CAD build for the part. Positions are in the model's coordinates, mm. Face numbers are marked on the shaded views. A direction names the side the tool comes from. Give positions to 0.01 mm unless a question says otherwise; leave off trailing zeros. Write each loop counter-clockwise with the first axis right and the second up, starting at its lowest first coordinate (ties: lowest second). Pieces come first, ordered by that corner, then holes. Notation, with made-up numbers: (-3.75, -26) - (23.25, -26) arc R16 ccw to (23.25, 5) - close; hole circle Ø9 at (6.25, 55). An arc over 180 degrees is marked (long way). Answer as a JSON object with one key per item and string values.
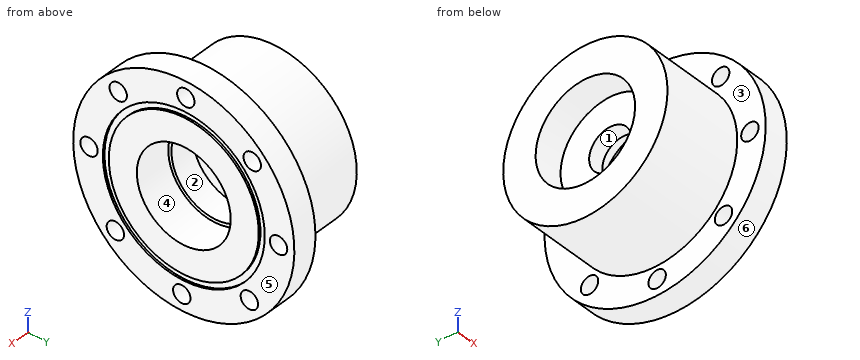
from build123d import *

# Parameters (mm, degrees)
M6_CLEARANCE_HOLE1_D = 7


with BuildPart() as part:
    # Main sketch → Revolve1 (revolve)
    with BuildSketch(Plane.XY, mode=Mode.PRIVATE) as revolve1_sk:
        Polygon((0, 8.500000018), (0, 20.000000005), (-11.999999876, 20.000000005), (-11.999999876, 33.02), (21.59, 33.02), (21.59, 44.45), (31.75, 44.45), (31.75, 32.54375), (30.972125, 32.54375), (30.972125, 30.1625), (31.75, 30.1625), (31.75, 18.8722), (16.6116, 18.8722), (16.6116, 17.6022), (6.35, 17.6022), (6.35, 8.500000018), align=None)
    revolve(revolve1_sk.sketch.rotate(Axis((71.950113838, 0, 0), (-1, 0, 0)), 90), axis=Axis((71.950113838, 0, 0), (-1, 0, 0)))

    # M6 Clearance Hole1 (through all)
    with Locations(Plane(origin=(31.75, 0, 0), x_dir=(0, 0, -1), z_dir=(1, 0, 0))):
        with Locations((0, 0), (-38.091322418, 0.813115257), (-27.509591698, -26.359673074), (-0.813115257, -38.091322418), (26.359673074, -27.509591698), (38.091322418, -0.813115257), (27.509591698, 26.359673074), (0.813115257, 38.091322418), (-26.359673074, 27.509591698)):
            Hole(M6_CLEARANCE_HOLE1_D / 2)


solid = part.part
Item 1: Which spindle directions (+Z, -Z, +X, -X, +Y, -Y) get a long thin tool onto all of the face, cutting with end or side? Do the marked faces 1, 2 and 3. Say none if no direction does.
Entries:
{"face 1": "+X, -X", "face 2": "+X", "face 3": "-X"}
Item 2: Cut at D-D (z = 14). Give the cut face in (x, y).
Entries:
{"outline": "(-12, -29.91) - (21.59, -29.91) - (21.59, -42.19) - (31.75, -42.19) - (31.75, -29.38) - (30.97, -29.38) - (30.97, -26.72) - (31.75, -26.72) - (31.75, -12.66) - (16.61, -12.66) - (16.61, -10.67) - (6.35, -10.67) - (6.35, 10.67) - (16.61, 10.67) - (16.61, 12.66) - (31.75, 12.66) - (31.75, 26.72) - (30.97, 26.72) - (30.97, 29.38) - (31.75, 29.38) - (31.75, 42.19) - (21.59, 42.19) - (21.59, 29.91) - (-12, 29.91) - (-12, 14.28) - (0, 14.28) - (0, -14.28) - (-12, -14.28) - close"}
Item 3: Cut at C-C (x = 23.5). State how many separate pieces and enclosed holes the cut face has, and give its area (3 significant figures).
Entries:
{"separate pieces": "1", "enclosed holes": "9", "area": "4,780 mm2"}
Item 4: Mould opens along Z. For the marked faces 4, 5 and 6 say: +Z half, -Z half, draft (parallel to the pull), parting line (faces both ways), or undercut.
Entries:
{"face 4": "undercut", "face 5": "draft", "face 6": "parting line"}
Item 5: Cut at A-A (z = 27). Give the cut face in (x, y).
Entries:
{"outline": "(-12, -19.01) - (21.59, -19.01) - (21.59, -22.9) - (31.75, -22.9) - (31.75, -18.17) - (30.97, -18.17) - (30.97, -13.45) - (31.75, -13.45) - (31.75, 13.45) - (30.97, 13.45) - (30.97, 18.17) - (31.75, 18.17) - (31.75, 24.07) - (21.59, 24.07) - (21.59, 19.01) - (-12, 19.01) - close; (21.59, -35.31) - (31.75, -35.31) - (31.75, -29.82) - (21.59, -29.82) - close; (21.59, 30.95) - (31.75, 30.95) - (31.75, 35.31) - (21.59, 35.31) - close"}
Item 6: Probe line 1 (Y direction, x = 3, z = 0); line 2 (Z direction, x = 25, y = 1.5); line 3 (X direction, y = 5, z = 13). List the from-to ranges inside material, lowest first. Write a range as from..to.
Entries:
{"line 1": "-33.02..-8.5, 8.5..33.02", "line 2": "-44.42..-40.72, -35.46..-18.81, 18.81..34.66, 41.52..44.42", "line 3": "0..6.35"}
Item 7: Cut at B-B (x = 12). Give the cut face in (y, z), and give its area (3 significant figures).
Entries:
{"outline": "circle Ø66.04 at (0, 0); hole circle Ø35.2 at (0, 0)", "area": "2,450 mm2"}
Item 8: Flat gauge pins, fed straight in: P1, Ø4, axis at y = -38.09, z = 0.81, coming from the -X side; P2, Ø3, axis at x = 24.5, z = -20.5, coming from the -Y side; P3, Ø19, axis at y = 0.5, z = -0.5, coming from the +X side; P4, Ø10, axis at x = 12, z = -10.5, coming from the -Y side. Where does each tip first touch, or does it go through?
Entries:
{"P1": "through", "P2": "y = -40.18", "P3": "x = 6.35", "P4": "y = -32.56"}
